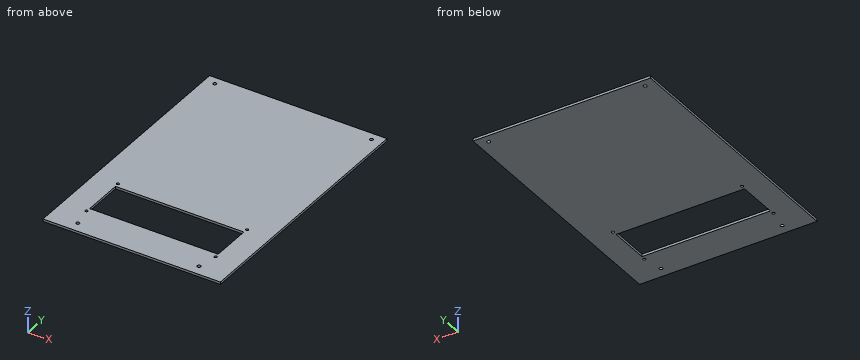
from build123d import *

# Parameters (mm, degrees)
SKETCH1_W                 = 221
SKETCH1_H                 = 323
BOSS_EXTRUDE1_DEPTH       = 3
SKETCH2_W                 = 160
SKETCH2_H                 = 50
CUT_EXTRUDE1_DEPTH        = 4
CUT_EXTRUDE2_REACH        = 5
SKETCH5_R                 = 1.7
F_4_0MM_DOWEL_HOLE1_D     = 4.2
F_4_0MM_DOWEL_HOLE1_DEPTH = 3


with BuildPart() as part:
    # Sketch1 → Boss-Extrude1 (new body)
    with BuildSketch(Plane(origin=(0, 0, -125.5), x_dir=(-1, 0, 0), z_dir=(0, 0, -1))):
        with Locations((0, 148.5)):
            Rectangle(SKETCH1_W, SKETCH1_H)
    extrude(amount=-BOSS_EXTRUDE1_DEPTH)

    # Sketch2 → Cut-Extrude1 (cut, through all)
    with BuildSketch(Plane.XY.offset(-122.5)):
        with Locations((0, 55)):
            Rectangle(SKETCH2_W, SKETCH2_H)
    extrude(amount=-CUT_EXTRUDE1_DEPTH, mode=Mode.SUBTRACT)

    # Sketch5 → Cut-Extrude2 (cut, up to next)
    with BuildSketch(Plane(origin=(0, 0, -125.5), x_dir=(-1, 0, 0), z_dir=(0, 0, -1)), mode=Mode.PRIVATE) as cut_extrude2_sk1:
        with Locations((80.5, 85.5)):
            Circle(SKETCH5_R)
    cut_extrude2_tool1 = extrude(cut_extrude2_sk1.sketch, amount=-CUT_EXTRUDE2_REACH, mode=Mode.PRIVATE) & part.part
    add(cut_extrude2_tool1.solids().sort_by_distance((-80.5, 85.5, -125.5))[0], mode=Mode.SUBTRACT)
    # Sketch5 → Cut-Extrude2 (cut, up to next)
    with BuildSketch(Plane(origin=(0, 0, -125.5), x_dir=(-1, 0, 0), z_dir=(0, 0, -1)), mode=Mode.PRIVATE) as cut_extrude2_sk2:
        with Locations((80.5, 24.5)):
            Circle(SKETCH5_R)
    cut_extrude2_tool2 = extrude(cut_extrude2_sk2.sketch, amount=-CUT_EXTRUDE2_REACH, mode=Mode.PRIVATE) & part.part
    add(cut_extrude2_tool2.solids().sort_by_distance((-80.5, 24.5, -125.5))[0], mode=Mode.SUBTRACT)
    # Sketch5 → Cut-Extrude2 (cut, up to next)
    with BuildSketch(Plane(origin=(0, 0, -125.5), x_dir=(-1, 0, 0), z_dir=(0, 0, -1)), mode=Mode.PRIVATE) as cut_extrude2_sk3:
        with Locations((-80.5, 24.5)):
            Circle(SKETCH5_R)
    cut_extrude2_tool3 = extrude(cut_extrude2_sk3.sketch, amount=-CUT_EXTRUDE2_REACH, mode=Mode.PRIVATE) & part.part
    add(cut_extrude2_tool3.solids().sort_by_distance((80.5, 24.5, -125.5))[0], mode=Mode.SUBTRACT)
    # Sketch5 → Cut-Extrude2 (cut, up to next)
    with BuildSketch(Plane(origin=(0, 0, -125.5), x_dir=(-1, 0, 0), z_dir=(0, 0, -1)), mode=Mode.PRIVATE) as cut_extrude2_sk4:
        with Locations((-80.5, 85.5)):
            Circle(SKETCH5_R)
    cut_extrude2_tool4 = extrude(cut_extrude2_sk4.sketch, amount=-CUT_EXTRUDE2_REACH, mode=Mode.PRIVATE) & part.part
    add(cut_extrude2_tool4.solids().sort_by_distance((80.5, 85.5, -125.5))[0], mode=Mode.SUBTRACT)

    # Ø4.0mm Dowel Hole1
    with Locations(Plane.XY.offset(-122.5)):
        with Locations((-97.5, 300), (97.5, 300), (75.5, 0), (-75.5, 0)):
            Hole(F_4_0MM_DOWEL_HOLE1_D / 2, depth=F_4_0MM_DOWEL_HOLE1_DEPTH)


solid = part.part
Source: CAD feature listing. Evaluate the final solid. Frame: model axes, mm. Give positions to 0.01 mm unless a question says otherwise; leave off trailing zeros. Order: outer loops, then holes, each group sorted by start corner. A loop starts at its lowest first (then second) coordinate and runs counter-clockwise, first axis right, second up. Notation, with made-up numbers: (-22, 47) -> (-7, 47) arc R27 cw to (-7, 64) -> close; hole circle Ø4 at (-12.5, 42). An arc over 180 degrees is marked (long way). Write item = value, one per line.
Item 1: Section query B-B (z = -124.5). State how many separate pieces and enclosed holes the cut face has, then the cut area to 3 significant figures.
Check result:
separate_pieces = 1
enclosed_holes = 9
area = 63,300 mm²
Item 2: Ray query, probe 1 along Y at (x, z) = (80.5, -123.45); probe 2 along Y at (x, z) = (60, -124.95). Return the intervals inside material, ascending.
Check result:
probe_1 = -13 to 22.8, 26.2 to 83.8, 87.2 to 310
probe_2 = -13 to 30, 80 to 310
Item 3: Section query A-A (x = -42.5). Output: boundary loops of the cut face in (y, z), then the cut area to 3 significant figures.
Check result:
outline = (-13, -125.5) -> (30, -125.5) -> (30, -122.5) -> (-13, -122.5) -> close; (80, -125.5) -> (310, -125.5) -> (310, -122.5) -> (80, -122.5) -> close
area = 819 mm²
